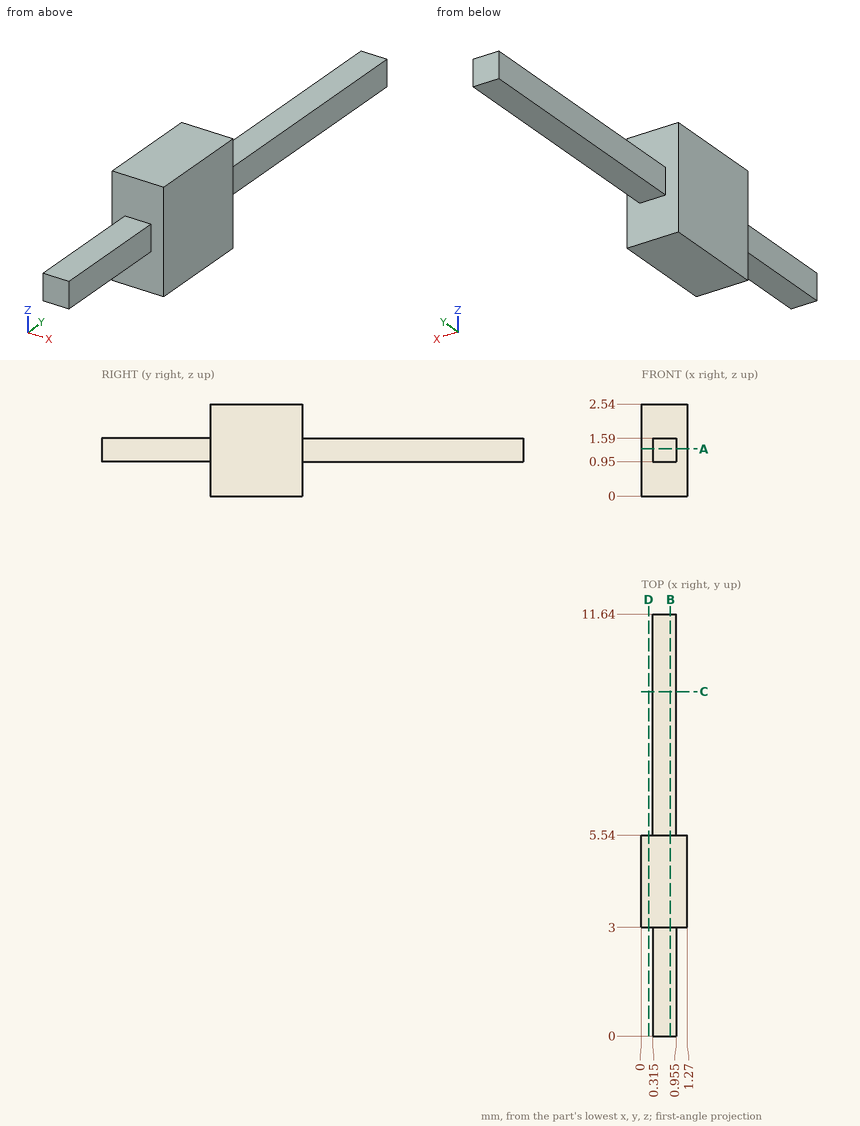
Answer from the drawing. Dimensions are ordinates in mm from the lowest x, y and z of the part. Give positions to 0.01 mm unless a question says otherwise; leave off trailing zeros. Loops run counter-clockwise (first coordinate to the right, second up) from the corner with the lowest first, then second, coordinate; pieces in that order, holes last. Notation, with made-up numbers: (83, 10.25) - (125, 10.25) arc R23 ccw to (125, 33.25) - close; hole circle Ø9 at (-30, 29.5). An arc over 180 degrees is marked (long way). Answer as a JSON object with one key per item and string values.
1. A cutting plane is placed at A-A (z = 1.3). Write down the section's boundary in (x, y) (3 decimals).
Determined:
{"outline": "(0, 3) - (0.315, 3) - (0.315, 0) - (0.955, 0) - (0.955, 3) - (1.27, 3) - (1.27, 5.54) - (0.955, 5.54) - (0.955, 11.64) - (0.315, 11.64) - (0.315, 5.54) - (0, 5.54) - close"}
2. Flat-ended cylindrical pins translate along their axes: pin 1 Ø0.7 at (y, z) = (9, 1) entering from -X (3 decimals); pin 2 Ø0.7 at (x, y) = (1, 2) entering from +Z; pin 3 Ø0.5 at (y, z) = (10, 1.5) entering from +X (3 decimals). Find the tip coordinate at first contact, or state that the pin passes through.
Determined:
{"pin 1": "x = 0.315", "pin 2": "z = 1.59", "pin 3": "x = 0.955"}
3. A cutting plane is placed at D-D (x = 0.2). Write down the section's boundary in (y, z).
Determined:
{"outline": "(3, 0) - (5.54, 0) - (5.54, 2.54) - (3, 2.54) - close"}
4. A cutting plane is placed at B-B (x = 0.8). Write down the section's boundary in (y, z).
Determined:
{"outline": "(0, 0.95) - (3, 0.95) - (3, 0) - (5.54, 0) - (5.54, 0.95) - (11.64, 0.95) - (11.64, 1.59) - (5.54, 1.59) - (5.54, 2.54) - (3, 2.54) - (3, 1.59) - (0, 1.59) - close"}
5. Find the intervals of material crossed by L1, parallel to Y at x = 0.1, z = 1.15; L2, parallel to X at y = 5.75, z = 1.1 (3 decimals); L3, parallel to Z at x = 0.9, y = 8, in increasing order. Write a range as [from, to].
Determined:
{"L1": "[3, 5.54]", "L2": "[0.315, 0.955]", "L3": "[0.95, 1.59]"}
6. A cutting plane is placed at C-C (y = 9.5). Write down the section's boundary in (x, z) (3 decimals), then the cut area to 3 significant figures.
Determined:
{"outline": "(0.315, 0.95) - (0.955, 0.95) - (0.955, 1.59) - (0.315, 1.59) - close", "area": "0.410 mm²"}
